Check sheet for the modelled part. Datum: model origin and axes. Units: mm. A direction names the side the tool comes from. Give positions to 0.01 mm unless a question says otherwise; leave off trailing zeros. Write each loop counter-clockwise with the first axis right and the second up, starting at its lowest first coordinate (ties: lowest second). Pieces come first, ordered by that corner, then holes. Notation, with made-up numbers: (64, 31.25) -> (111, 31.25) arc R29 cw to (111, 51.25) -> close; hole circle Ø7 at (9, 54). An arc over 180 degrees is marked (long way). Return JSON: item names as keys, results as strings.
from build123d import *

# Parameters (mm, degrees)
SKETCH1_R           = 7
BOSS_EXTRUDE1_DEPTH = 1
SKETCH2_W           = 5
SKETCH2_H           = 1
BOSS_EXTRUDE2_DEPTH = 2
SKETCH3_W           = 0.5
SKETCH3_H           = 0.452823542
BOSS_EXTRUDE3_DEPTH = 3
DRAFT9_ANGLE        = 1


with BuildPart() as part:
    # Sketch1 → Boss-Extrude1 (new body)
    with BuildSketch(Plane.XY):
        Circle(SKETCH1_R)
    extrude(amount=BOSS_EXTRUDE1_DEPTH)

    # Sketch2 → Boss-Extrude2 (add)
    with BuildSketch(Plane(origin=(0, 0, 0), x_dir=(-1, 0, 0), z_dir=(0, 0, -1))):
        with Locations((-0.154644107, 3.992933826)):
            Rectangle(SKETCH2_W, SKETCH2_H)
    extrude(amount=BOSS_EXTRUDE2_DEPTH)

    # Sketch3 → Boss-Extrude3 (add)
    with BuildSketch(Plane(origin=(0, 4.492933826, 0), x_dir=(1, 0, 0), z_dir=(0, 1, 0))):
        with Locations((1.154644107, 0.365882794)):
            Rectangle(SKETCH3_W, SKETCH3_H)
        with Locations((2.154644107, 0.365882794)):
            Rectangle(SKETCH3_W, SKETCH3_H)
        with Locations((0.154644107, 0.365882794)):
            Rectangle(SKETCH3_W, SKETCH3_H)
        with Locations((-0.845355893, 0.365882794)):
            Rectangle(SKETCH3_W, SKETCH3_H)
        with Locations((-1.845355893, 0.365882794)):
            Rectangle(SKETCH3_W, SKETCH3_H)
    extrude(amount=BOSS_EXTRUDE3_DEPTH)

    # Draft9
    draft9_faces = [part.faces().sort_by_distance(p)[0] for p in [
        (2.404644107, 5.992933826, -0.365882794),
    ]]
    draft(draft9_faces, Plane.ZX.offset(7.492933826), DRAFT9_ANGLE)


solid = part.part
(1) Depth check by flat-ended pin: pin 1 Ø0.5 at (y, z) = (6, -0.5) entering from -X; pin 2 Ø1.6 at (x, z) = (1, -1) entering from -Y; pin 3 Ø0.8 at (y, z) = (4, -1) entering from +X. Enter the tip coordinate at first touch or a pass-through.
Reply:
{"pin 1": "x = -2.1", "pin 2": "y = 3.49", "pin 3": "x = 2.65"}
(2) Cross-section at B-B on z = 0.75. Enter the section's corners in (x, y), then the cut area to 3 significant figures.
Reply:
{"outline": "circle Ø14 at (0, 0)", "area": "154 mm^2"}
(3) Cross-section at D-D on z = -1.35. Enter the section's corners in (x, y), then the cut area to 3 significant figures.
Reply:
{"outline": "(-2.35, 3.49) -> (2.65, 3.49) -> (2.65, 4.49) -> (-2.35, 4.49) -> close", "area": "5.00 mm^2"}
(4) Cross-section at A-A on y = 5. Enter the section's corners in (x, z), then the cut area to 3 significant figures.
Reply:
{"outline": "(-4.9, 0) -> (4.9, 0) -> (4.9, 1) -> (-4.9, 1) -> close; (-2.1, -0.59) -> (-1.6, -0.59) -> (-1.6, -0.14) -> (-2.1, -0.14) -> close; (-1.1, -0.59) -> (-0.6, -0.59) -> (-0.6, -0.14) -> (-1.1, -0.14) -> close; (-0.1, -0.59) -> (0.4, -0.59) -> (0.4, -0.14) -> (-0.1, -0.14) -> close; (0.9, -0.59) -> (1.4, -0.59) -> (1.4, -0.14) -> (0.9, -0.14) -> close; (1.9, -0.59) -> (2.45, -0.59) -> (2.45, -0.14) -> (1.9, -0.14) -> close", "area": "10.9 mm^2"}
(5) Cross-section at C-C on y = 0. Enter the section's corners in (x, z), then the cut area to 3 significant figures.
Reply:
{"outline": "(-7, 0) -> (7, 0) -> (7, 1) -> (-7, 1) -> close", "area": "14.0 mm^2"}
(6) Release check for a two-part mould opening along Y. For faces 4 (the flat face through (0, 3.493, -1)), 5 (the flat face through (0, 0, 1)), 6 (the cylindrical face through (6.466, -2.681, 0.493)) record: pulls with the +Y half, pulls with the -Y half, needs draft (parallel to the pull), parting line crosses it, or undercut.
Reply:
{"face 4": "pulls with the -Y half", "face 5": "needs draft", "face 6": "parting line crosses it"}
(7) Set-up check for faces 1 (the flat face through (0, 4, -2)), 2 (the flat face through (-2.345, 4, -1)), 3 (the flat face through (2.655, 4, -1)): record each of +Z, -Z, +X, -X, +Y, -Y from which the full face is reachable in a straight line by a thin tool's end or side.
Reply:
{"face 1": "-Z, +X, -X, +Y, -Y", "face 2": "-Z, -X, +Y, -Y", "face 3": "-Z, +X, +Y, -Y"}
(8) Thickness scan on L1, parallel to Z at x = 5, y = 0; L2, parallel to Y at x = 1, z = -0.75; L3, parallel to Y at x = -2.5, z = 0.7. Record the ranges inside material, lowest first.
Reply:
{"L1": "0 to 1", "L2": "3.49 to 4.49", "L3": "-6.54 to 6.54"}
